```python
from build123d import *

# Parameters (mm, degrees)
SKETCH1_W           = 76.2
SKETCH1_H           = 50.8
BOSS_EXTRUDE1_DEPTH = 9.398
CUT_EXTRUDE1_DEPTH  = 9.398
SKETCH4_R           = 12.7
SKETCH4_R_2         = 3.429
BOSS_EXTRUDE2_DEPTH = 25.4


with BuildPart() as part:
    # Sketch1 → Boss-Extrude1 (new body)
    with BuildSketch(Plane(origin=(0, 0, 0), x_dir=(1, 0, 0), z_dir=(0, 1, 0))):
        with Locations((38.1, 25.4)):
            Rectangle(SKETCH1_W, SKETCH1_H)
    extrude(amount=BOSS_EXTRUDE1_DEPTH)

    # Sketch3 → Cut-Extrude1 (cut)
    with BuildSketch(Plane(origin=(0, 9.398, 0), x_dir=(1, 0, 0), z_dir=(0, 1, 0))):
        with BuildLine():
            Line((8.636, 43.434), (8.636, 7.366))
            ThreePointArc((8.636, 7.366), (12.7, 3.302), (16.764, 7.366))
            Line((16.764, 7.366), (16.764, 43.434))
            ThreePointArc((16.764, 43.434), (12.7, 47.498), (8.636, 43.434))
        make_face()
        with BuildLine():
            Line((67.564, 43.434), (67.564, 7.366))
            ThreePointArc((67.564, 7.366), (63.5, 3.302), (59.436, 7.366))
            Line((59.436, 7.366), (59.436, 43.434))
            ThreePointArc((59.436, 43.434), (63.5, 47.498), (67.564, 43.434))
        make_face()
    extrude(amount=-CUT_EXTRUDE1_DEPTH, mode=Mode.SUBTRACT)

    # Sketch4 → Boss-Extrude2 (add)
    with BuildSketch(Plane(origin=(0, 9.398, 0), x_dir=(1, 0, 0), z_dir=(0, 1, 0))):
        with Locations(Location((38.1, 25.4, 0), (0, 0, 270))):
            Circle(SKETCH4_R)
        with Locations(Location((38.1, 25.4, 0), (0, 0, 270))):
            Circle(SKETCH4_R_2, mode=Mode.SUBTRACT)
    extrude(amount=BOSS_EXTRUDE2_DEPTH)


solid = part.part
```
The model under review builds one solid part; all positions refer to its coordinate system, in mm. A direction names the side the tool comes from. Round coordinates to 2 decimals unless told otherwise and drop trailing zeros. Write each loop counter-clockwise with the first axis right and the second up, starting at its lowest first coordinate (ties: lowest second). Pieces come first, ordered by that corner, then holes.
(1) Machinability: for faces 4 (the cylindrical face through (39.13, 21.92, -22.13)), 5 (the flat face through (76.2, 5, -25)), 6 (the cylindrical face through (63.589, 4.765, -3.303)), which of the approach directions +Z, -Z, +X, -X, +Y, -Y give a long, thin tool a straight path to every point of the face, cutting with its end or side? Answer none if there is none.
(2) We need section B-B on z = -25.4. Give the boundary of the cut face in (x, y).
(3) We need section D-D on x = 38.1. Give the boundary of the cut face in (y, z), and give its area (3 significant figures).
(4) Mouldability with a two-part tool opening along X and no side actions: class faces 1 (the cylindrical face through (63.411, 4.765, -47.497)), 2 (the flat face through (29, 9.398, -14)), 3 (the cylindrical face through (48.809, 21.92, -18.573)) as +X half, -X half, draft (parallel to the pull), parting line (faces both ways), or undercut.
(5) We need section C-C on y = 7. Give the boundary of the cut face in (x, z), and give its area (3 significant figures).
(6) Wall thickness on L1, parallel to X at y = 3, z = -11; L2, parallel to Z at x = 38, y = 29; L3, parallel to Y at x = 26.5, z = -47: over which ranges is each line inside the solid? List them lowest first.
(7) Insertion check: pin 1 (2 mm diameter, centred on x = 14.5, z = -24.5, fed in from +Y); pin 2 (1.5 mm diameter, centred on y = 25.5, z = -20, fed in from +X); pin 3 (3.5 mm diameter, centred on x = 37, z = -26.5, fed in from +Y). Each pin has a flat end and moves straight along its axis. Give the tip position at first contact, or say it passes through.
(8) We need section A-A on x = 12.7. Give the boundary of the cut face in (y, z), and give its area (3 significant figures).
Findings below:
1. face 4: +Y
1. face 5: +Z, -Z, +X, +Y, -Y
1. face 6: +Y, -Y
2. outline: (0, 0) - (8.64, 0) - (8.64, 9.4) - (0, 9.4) - close; (16.76, 0) - (59.44, 0) - (59.44, 9.4) - (50.8, 9.4) - (50.8, 34.8) - (41.53, 34.8) - (41.53, 9.4) - (34.67, 9.4) - (34.67, 34.8) - (25.4, 34.8) - (25.4, 9.4) - (16.76, 9.4) - close; (67.56, 0) - (76.2, 0) - (76.2, 9.4) - (67.56, 9.4) - close
3. outline: (0, -50.8) - (9.4, -50.8) - (9.4, -38.1) - (34.8, -38.1) - (34.8, -28.83) - (9.4, -28.83) - (9.4, -21.97) - (34.8, -21.97) - (34.8, -12.7) - (9.4, -12.7) - (9.4, 0) - (0, 0) - close
3. area: 948 mm2
4. face 1: undercut
4. face 2: draft
4. face 3: parting line
5. outline: (0, -50.8) - (76.2, -50.8) - (76.2, 0) - (0, 0) - close; hole (8.64, -43.43) arc R4.06 ccw to (16.76, -43.43) - (16.76, -7.37) arc R4.06 ccw to (8.64, -7.37) - close; hole (59.44, -43.43) arc R4.06 ccw to (67.56, -43.43) - (67.56, -7.37) arc R4.06 ccw to (59.44, -7.37) - close
5. area: 3,180 mm2
6. L1: x = 0 to 8.64, 16.76 to 59.44, 67.56 to 76.2
6. L2: z = -38.1 to -28.83, -21.97 to -12.7
6. L3: y = 0 to 9.4
7. pin 1: passes through
7. pin 2: stops at x = 49.92
7. pin 3: stops at y = 9.4
8. outline: (0, -50.8) - (9.4, -50.8) - (9.4, -47.5) - (0, -47.5) - close; (0, -3.3) - (9.4, -3.3) - (9.4, 0) - (0, 0) - close
8. area: 62.1 mm2
